Autodesk Inventor part; units mm, degrees
ref_plane "YZ Plane" through (0, 0, 0) normal (1, 0, 0) x (0, 1, 0)
ref_plane "XZ Plane" through (0, 0, 0) normal (0, 1, 0) x (-1, 0, 0)
ref_plane "XY Plane" through (0, 0, 0) normal (0, 0, 1) x (1, 0, 0)
sketch "Náčrt1" plane through (0, 0, 0) normal (0, 0, 1) x (1, 0, 0)
  line L0 (0, 35) -> (0, -35)
  line L1 (-63, 0) -> (63, 0)
  line L2 (-45, 25) -> (45, 25)
  line L3 (45, 25) -> (45, -25)
  line L4 (45, -25) -> (-45, -25)
  line L5 (-45, -25) -> (-45, 25)
  point P0 (0, 0)
  dimension "d0" = 90
  dimension "d1" = 50
extrude "Vysunutí1" add sketch "Náčrt1" along normal blind 5
sketch "Náčrt4" plane through (0, 0, 0) normal (0, 0, -1) x (-1, 0, 0)
  line L0 (45, 25) -> (45, -25)
  line L1 (-45, 25) -> (45, 25)
  line L2 (-45, -25) -> (-45, 25)
  line L3 (45, -25) -> (-45, -25)
  line L4 (0, -35) -> (0, 35)
  line L5 (-63, 0) -> (63, 0)
  point P0 (0, 0)
  point P1 (-39.5, 19.5)
  dimension "d13" = 5.5
  dimension "d14" = 5.5
hole "Díra1" at (39.5, 19.5, 0) direction (0, 0, 1) diameter 3.4 end through all counterbore diameter 6.1 counterbore depth 3
mirror "Zrcadlit2" about plane through (0, 0, 0) normal (0, 1, 0) of "Díra1"
mirror "Zrcadlit3" about plane through (0, 0, 0) normal (1, 0, 0) of "Díra1", "Zrcadlit2"
fillet "Zaoblení2" radius 2 8 edges at (0, 25, 0) (45, 0, 0) (45, 25, 2.5) (0, -25, 0) (45, -25, 2.5) (-45, 0, 0) (-45, -25, 2.5) (-45, 25, 2.5)
sketch "Náčrt6" plane through (0, 0, 0) normal (0, 0, -1) x (-1, 0, 0)
  circle A0 centre (-39.5, 19.5) radius 3.05
  circle A1 centre (-39.5, -19.5) radius 3.05
  circle A2 centre (39.5, 19.5) radius 3.05
  circle A3 centre (39.5, -19.5) radius 3.05
  line L0 (43, -23) -> (-43, -23)
  line L1 (43, 23) -> (43, -23)
  line L2 (-43, 23) -> (43, 23)
  line L3 (-43, -23) -> (-43, 23)
  line L4 (-43, 23) -> (-45, 23)
  line L5 (-45, 23) -> (-45, -23)
  line L6 (-45, -23) -> (-43, -23)
  line L7 (-43, -23) -> (-43, 23)
  line L8 (-45, 3.75) -> (-36, 3.75)
  line L9 (-36, 3.75) -> (-36, -3.75)
  line L10 (-36, -3.75) -> (-45, -3.75)
  line L11 (-45, -3.75) -> (-45, 3.75)
  line L12 (-63, 0) -> (63, 0)
  point P0 (0, 0)
  dimension "d23" = 9
  dimension "d24" = 7.5
extrude "Vysunutí4" cut sketch "Náčrt6" against normal through all contours L10 L5 L12 L3 | L3 L12 L9 L10 | L12 L3 L8 L9 | L12 L5 L8 L3
mirror "Zrcadlit4" about plane through (0, 0, 0) normal (1, 0, 0) of "Vysunutí4"
properties part number "tcs3200_gate_lid_3D tisk"
The listing builds one solid part. Answer for the finished solid, in the listing's coordinates (mm). A direction names the side the tool comes from. Round coordinates to 2 decimals unless told otherwise and drop trailing zeros. Order: outer loops, then holes, each group sorted by start corner. A loop starts at its lowest first (then second) coordinate and runs counter-clockwise, first axis right, second up. Notation, with made-up numbers: (26.25, 33) - (49.25, 33) arc R21 ccw to (49.25, 46) - close; hole circle Ø7 at (-16, 27.25). An arc over 180 degrees is marked (long way). Put each result on its own line as item: value. Start each with the question number.
(1) Find section A-A (y = 19.5). Give the vertices of the cut face in (x, z).
(2) Straight lines are drawn through the part: probe 1 along Y at (x, z) = (39.5, 2.25); probe 2 along X at (y, z) = (19.5, 4.45); probe 3 along X at (y, z) = (19.5, 2.1). For each, find the intervals that lie inside material, in ascending order. Write a range as from..to.
(3) Find section C-C (z = 1.2). Give the vertices of the cut face in (x, y).
(4) For faces 1 (the cylindrical face through (36.523, -18.839, 1.521)), 2 (the flat face through (41, 3.75, 2)), 3 (the flat face through (-41, -3.75, 2)), determine the directions among +Z, -Z, +X, -X, +Y, -Y from which every point of the face is accessible in a straight line to the end or side of a thin tool.
(5) Given P1, Ø5.5, axis at x = -39.5, y = -19.5, coming from the +Z side; P2, Ø4, axis at x = -39.5, y = 19.5, coming from the -Z side, each flat-ended and moving along its own axis, determine where each tip first touches the part or whether it passes through.
(6) Find section B-B (x = 39.5). Give the vertices of the cut face in (y, z).
(7) Determine the mould class of faces 4 (the flat face through (-45, 13, 3)), 5 (the flat face through (36, 0, 2)), 6 (the cylindrical face through (42.477, 18.839, 1.521)) for opening direction X: released by +X, released by -X, zero draft, split by the parting line, or undercut.
(8) Find section D-D (y = -1.5). Give the vertices of the cut face in (x, z).
Reply:
1. outline: (-45, 2) arc R2 ccw to (-43, 0) - (-42.55, 0) - (-42.55, 3) - (-41.2, 3) - (-41.2, 5) - (-45, 5) - close; (-37.8, 3) - (-36.45, 3) - (-36.45, 0) - (36.45, 0) - (36.45, 3) - (37.8, 3) - (37.8, 5) - (-37.8, 5) - close; (41.2, 3) - (42.55, 3) - (42.55, 0) - (43, 0) arc R2 ccw to (45, 2) - (45, 5) - (41.2, 5) - close
2. probe 1: -25..-22.55, -16.45..-3.75, 3.75..16.45, 22.55..25
2. probe 2: -45..-41.2, -37.8..37.8, 41.2..45
2. probe 3: -45..-42.55, -36.45..36.45, 42.55..45
3. outline: (-44.83, -23) arc R1.83 ccw to (-43, -24.83) - (43, -24.83) arc R1.83 ccw to (44.83, -23) - (44.83, -3.75) - (36, -3.75) - (36, 3.75) - (44.83, 3.75) - (44.83, 23) arc R1.83 ccw to (43, 24.83) - (-43, 24.83) arc R1.83 ccw to (-44.83, 23) - (-44.83, 3.75) - (-36, 3.75) - (-36, -3.75) - (-44.83, -3.75) - close; hole circle Ø6.1 at (-39.5, -19.5); hole circle Ø6.1 at (-39.5, 19.5); hole circle Ø6.1 at (39.5, -19.5); hole circle Ø6.1 at (39.5, 19.5)
4. face 1: -Z
4. face 2: +Z, -Z, +X
4. face 3: +Z, -Z, -X
5. P1: z = 5
5. P2: z = 3
6. outline: (-25, 2) arc R2 ccw to (-23, 0) - (-22.55, 0) - (-22.55, 3) - (-21.2, 3) - (-21.2, 5) - (-25, 5) - close; (-17.8, 3) - (-16.45, 3) - (-16.45, 0) - (-3.75, 0) - (-3.75, 5) - (-17.8, 5) - close; (3.75, 0) - (16.45, 0) - (16.45, 3) - (17.8, 3) - (17.8, 5) - (3.75, 5) - close; (21.2, 3) - (22.55, 3) - (22.55, 0) - (23, 0) arc R2 ccw to (25, 2) - (25, 5) - (21.2, 5) - close
7. face 4: released by -X
7. face 5: released by +X
7. face 6: undercut
8. outline: (-36, 0) - (36, 0) - (36, 5) - (-36, 5) - close
